Geometry check sheet. Reference: the model listing, model coordinates, mm. Round coordinates to 2 decimals unless told otherwise and drop trailing zeros. Write each loop counter-clockwise with the first axis right and the second up, starting at its lowest first coordinate (ties: lowest second). Pieces come first, ordered by that corner, then holes. Notation, with made-up numbers: M 51,4.5 L 57,4.5 A36 ccw 57,38.5 Z; hole C 6.5,44.5 d10. An arc over 180 degrees is marked long. Put each result on its own line as item: value. Start each with the question number.
(1) Gauge pin test, flat end, axial feed: pin 1 (3 mm diameter, centred on x = -15.5, y = -15.5, fed in from -Z). Record the tip position at first contact, or that the pin passes through.
(2) Section check A-A on y = 3. Record the cut outline in (x, z), then the cut area to 3 significant figures.
(3) Material ranges on probe 1 along Y at (x, z) = (-15.5, 4); probe 2 along X at (y, z) = (-15, 3.75); probe 3 along X at (y, z) = (-1, 5.5), recorded low to high.
(4) Section check B-B on x = -4. Record the cut outline in (y, z).
(5) Section check C-C on z = 8. Record the cut outline in (x, y).
(6) Mould release check, pull along X, two halves, no side actions. Record for faces 1 (the flat face through (-37.5, -5, 5)), 2 (the cylindrical face through (-14.6, 17, 5.1)), 3 (the flat face through (-1, -10, 0)): pulls with the +X half, pulls with the -X half, needs draft (parallel to the pull), parting line crosses it, or undercut.
from build123d import *

# Parameters (mm, degrees)
SKETCH1_W                  = 75
SKETCH1_H                  = 40
SKETCH1_R                  = 5
BOSS_EXTRUDE1_DEPTH        = 10
F_3_5_3_5_DIAMETER_HOLE1_D = 3.5
SKETCH4_W                  = 75
SKETCH4_H                  = 10
BOSS_EXTRUDE2_DEPTH        = 10


with BuildPart() as part:
    # Sketch1 → Boss-Extrude1 (new body)
    with BuildSketch(Plane.XY):
        Rectangle(SKETCH1_W, SKETCH1_H)
        Circle(SKETCH1_R, mode=Mode.SUBTRACT)
    extrude(amount=BOSS_EXTRUDE1_DEPTH)

    # Ø3.5 (3.5) Diameter Hole1 (through all)
    with Locations(Plane(origin=(0, 0, 0), x_dir=(-1, 0, 0), z_dir=(0, 0, -1))):
        with Locations((15.5, 15.5), (-15.5, 15.5), (-15.5, -15.5), (15.5, -15.5)):
            Hole(F_3_5_3_5_DIAMETER_HOLE1_D / 2)

    # Sketch4 → Boss-Extrude2 (add)
    with BuildSketch(Plane.XZ.offset(20)):
        with Locations((0, 5)):
            Rectangle(SKETCH4_W, SKETCH4_H)
    extrude(amount=BOSS_EXTRUDE2_DEPTH)


solid = part.part
Answers follow:
1. pin 1: passes through
2. outline: M -37.5,0 L -4,0 L -4,10 L -37.5,10 Z; M 4,0 L 37.5,0 L 37.5,10 L 4,10 Z
2. area: 670 mm^2
3. probe 1: y = -30 to -17.25, -13.75 to 13.75, 17.25 to 20
3. probe 2: x = -37.5 to -17.18, -13.82 to 13.82, 17.18 to 37.5
3. probe 3: x = -37.5 to -4.9, 4.9 to 37.5
4. outline: M -30,0 L -3,0 L -3,10 L -30,10 Z; M 3,0 L 20,0 L 20,10 L 3,10 Z
5. outline: M -37.5,-30 L 37.5,-30 L 37.5,20 L -37.5,20 Z; hole C -15.5,-15.5 d3.5; hole C -15.5,15.5 d3.5; hole C 0,0 d10; hole C 15.5,-15.5 d3.5; hole C 15.5,15.5 d3.5
6. face 1: pulls with the -X half
6. face 2: undercut
6. face 3: needs draft
